Design review of the part built by this model. Coordinates are the model's own, in mm. A direction names the side the tool comes from. Coordinates: 2 decimals unless noted, no trailing zeros. Write each loop counter-clockwise with the first axis right and the second up, starting at its lowest first coordinate (ties: lowest second). Pieces come first, ordered by that corner, then holes. Notation, with made-up numbers: (75, -9.75) -> (134, -9.75) arc R26 cw to (134, 9.25) -> close; hole circle Ø6 at (-10.75, -12). An arc over 180 degrees is marked (long way). Return JSON: item names as keys, results as strings. Group by question number.
Autodesk Inventor part; units mm, degrees
ref_plane "YZ Plane" through (0, 0, 0) normal (1, 0, 0) x (0, 1, 0)
ref_plane "XZ Plane" through (0, 0, 0) normal (0, 1, 0) x (-1, 0, 0)
ref_plane "XY Plane" through (0, 0, 0) normal (0, 0, 1) x (1, 0, 0)
sketch "Sketch1" plane through (0, 0, 0) normal (0, 0, 1) x (1, 0, 0)
  line L0 (-43, 17) -> (43, 17)
  line L1 (43, 17) -> (43, -25)
  line L2 (43, -25) -> (-43, -25)
  line L3 (-43, -25) -> (-43, 17)
  circle A0 centre (-37, 10) radius 2.5
  circle A1 centre (-37, -10) radius 2.5
  line L4 (0, 17) -> (0, -25) construction
  circle A2 centre (37, 10) radius 2.5
  circle A3 centre (37, -10) radius 2.5
  circle A4 centre (-9.5, -10) radius 2
  point P0 (0, 0)
  point P1 (-43, -4)
  dimension "d0" = 86
  dimension "d1" = 42
  dimension "d2" = 5
  dimension "d3" = 7
  dimension "d4" = 6
  dimension "d5" = 6
  dimension "d6" = 15
  dimension "d7" = 4
  dimension "d8" = 27.5
extrude "Extrusion3" add sketch "Sketch1" along normal blind 3.175
sketch "Sketch3" plane through (0, 0, 3.175) normal (0, 0, 1) x (1, 0, 0)
  line L0 (-25, 17) -> (25, 17)
  line L1 (25, 17) -> (25, 0)
  line L2 (25, 0) -> (-25, 0)
  line L3 (-25, 0) -> (-25, 17)
  line L4 (43, 17) -> (-43, 17)
  circle A0 centre (-9.5, -10) radius 2
  line L5 (25, 0) -> (0, 0)
  line L6 (0, 0) -> (0, -15)
  line L7 (0, -15) -> (25, -15)
  line L8 (25, -15) -> (25, 0)
  line L9 (-43, -25) -> (43, -25)
  point P0 (0, 0)
  point P1 (0, 17)
  dimension "d20" = 50
  dimension "d22" = 10
  dimension "d23" = 9.5
  dimension "d24" = 10
extrude "Extrusion4" cut sketch "Sketch3" against normal through all contours L0 L1 L2 L3 | L8 L7 L6 L2
equation "\"d5\" = d4"
equation "\"d24\" = d22"
properties part number "BaseAluminio"
Q1. Wall thickness on L1, parallel to Y at x = 37, z = 2.1; L2, parallel to X at y = -1, z = 1.4; L3, parallel to Y at x = 38, z = 2.55: over which ranges is each line inside the solid? List them lowest first.
Q2. We need section B-B on y = 10. Write out the cut boundary in (x, z) (3 decimals), plus the area to 4 significant figures.
Q3. We need section D-D on x = -9.5. Write out the cut boundary in (y, z) (3 decimals), plus the area to 3 significant figures.
Q4. The part is to be moulded in two halves that separate along X. For faces 3 (the flat face through (43, -4, 2)), 4 (the flat face through (-1, -8, 0)), 5 (the flat face through (25, 1, 2)), say which applies: +X half, -X half, draft (parallel to the pull), parting line (faces both ways), or undercut.
Q5. For faces 1 (the flat face through (34, 17, 2)), 2 (the flat face through (-12, 0, 2)), list the 3-axis set-ups (+Z, -Z, +X, -X, +Y, -Y) from which the entire face can be reached by the end or side of a thin tool; tool diameter is ignored.
Q6. We need section A-A on x = -37. Write out the cut boundary in (y, z) (3 decimals).
Q7. We need section C-C on z = 1.8. Write out the cut boundary in (x, y), plus the area to 3 significant figures.
Findings below:
{
 "1": {"L1": "y = -25 to -12.5, -7.5 to 7.5, 12.5 to 17", "L2": "x = -43 to 0, 25 to 43", "L3": "y = -25 to -12.29, -7.71 to 7.71, 12.29 to 17"},
 "2": {"outline": "(-43, 0) -> (-39.5, 0) -> (-39.5, 3.175) -> (-43, 3.175) -> close; (-34.5, 0) -> (-25, 0) -> (-25, 3.175) -> (-34.5, 3.175) -> close; (25, 0) -> (34.5, 0) -> (34.5, 3.175) -> (25, 3.175) -> close; (39.5, 0) -> (43, 0) -> (43, 3.175) -> (39.5, 3.175) -> close", "area": "82.55 mm^2"},
 "3": {"outline": "(-25, 0) -> (-12, 0) -> (-12, 3.175) -> (-25, 3.175) -> close; (-8, 0) -> (0, 0) -> (0, 3.175) -> (-8, 3.175) -> close", "area": "66.7 mm^2"},
 "4": {"face 3": "+X half", "face 4": "draft", "face 5": "undercut"},
 "5": {"face 1": "+Z, -Z, +X, -X, +Y", "face 2": "+Z, -Z, +Y"},
 "6": {"outline": "(-25, 0) -> (-12.5, 0) -> (-12.5, 3.175) -> (-25, 3.175) -> close; (-7.5, 0) -> (7.5, 0) -> (7.5, 3.175) -> (-7.5, 3.175) -> close; (12.5, 0) -> (17, 0) -> (17, 3.175) -> (12.5, 3.175) -> close"},
 "7": {"outline": "(-43, -25) -> (43, -25) -> (43, 17) -> (25, 17) -> (25, -15) -> (0, -15) -> (0, 0) -> (-25, 0) -> (-25, 17) -> (-43, 17) -> close; hole circle Ø5 at (-37, -10); hole circle Ø5 at (-37, 10); hole circle Ø4 at (-9.5, -10); hole circle Ø5 at (37, -10); hole circle Ø5 at (37, 10)", "area": "2,300 mm^2"}
}
